The model under review builds one solid part; all positions refer to its coordinate system, in mm. Round coordinates to 2 decimals unless told otherwise and drop trailing zeros. Loops run counter-clockwise (first coordinate to the right, second up) from the corner with the lowest first, then second, coordinate; pieces in that order, holes last. Notation, with made-up numbers: (64.25, -1.5) -> (120.25, -1.5) arc R4 ccw to (120.25, 3.5) -> close; hole circle Ø2 at (14.25, 0.25). An arc over 180 degrees is marked (long way). Use a Markdown table: item, result. Add a question column.
1) Consider section A-A on z = -14.5. Give the boundary of the cut face in (x, y).
2) Consider section D-D on y = 0.4. Give the boundary of the cut face in (x, z), plus the area to 3 significant figures.
3) Consider section B-B on x = 13. Give the boundary of the cut face in (y, z).
4) Mouldability with a two-part tool opening along Z and no side actions: class faces 1 (the cylindrical face through (55.066, 1.014, -33.683)), 2 (the flat face through (17, 2, -28)) as released by +Z, released by -Z, zero draft, split by the parting line, or undercut.
5) Consider section C-C on z = 0. Give the boundary of the cut face in (x, y), plus the area to 3 significant figures.
6) Wall thickness on probe 1 along X at (y, z) = (0.4, 0); probe 2 along Z at (x, y) = (-16, 1); probe 3 along X at (y, z) = (0.55, -16.5): over which ranges is each line inside the solid? List them lowest first.
from build123d import *

# Parameters (mm, degrees)
SKETCH1_W           = 118
SKETCH1_H           = 82
BOSS_EXTRUDE1_DEPTH = 2
SKETCH2_R           = 2.45
SKETCH2_W           = 95.88
SKETCH2_H           = 65.51
SKETCH2_W_2         = 12.69
SKETCH2_H_2         = 6.85
CUT_EXTRUDE4_DEPTH  = 10
SKETCH3_R           = 1.5
CUT_EXTRUDE7_DEPTH  = 10


with BuildPart() as part:
    # Sketch1 → Boss-Extrude1 (new body)
    with BuildSketch(Plane(origin=(0, 0, 0), x_dir=(1, 0, 0), z_dir=(0, 1, 0))):
        Rectangle(SKETCH1_W, SKETCH1_H)
    extrude(amount=BOSS_EXTRUDE1_DEPTH)

    # Sketch2 → Cut-Extrude4 (cut)
    with BuildSketch(Plane(origin=(0, 2, 0), x_dir=(1, 0, 0), z_dir=(0, 1, 0))):
        with Locations(Location((53, 35, 0), (0, 0, 270))):
            Circle(SKETCH2_R)
        with Locations((-6.06, -6.245)):
            Rectangle(SKETCH2_W, SKETCH2_H)
        with Locations((-47.655, 34.575)):
            Rectangle(SKETCH2_W_2, SKETCH2_H_2)
    extrude(amount=-CUT_EXTRUDE4_DEPTH, mode=Mode.SUBTRACT)

    # Sketch3 → Cut-Extrude7 (cut)
    with BuildSketch(Plane(origin=(0, 2, 0), x_dir=(1, 0, 0), z_dir=(0, 1, 0))):
        with Locations(Location((57, 0, 0), (0, 0, 270))):
            Circle(SKETCH3_R)
        with Locations(Location((-57, 0, 0), (0, 0, 270))):
            Circle(SKETCH3_R)
    extrude(amount=-CUT_EXTRUDE7_DEPTH, mode=Mode.SUBTRACT)


solid = part.part
Result set:
| question | item | result |
|---|---|---|
| 1 | outline | (-59, 0) -> (-54, 0) -> (-54, 2) -> (-59, 2) -> close; (41.88, 0) -> (59, 0) -> (59, 2) -> (41.88, 2) -> close |
| 2 | outline | (-59, -41) -> (59, -41) -> (59, 41) -> (-59, 41) -> close; hole circle Ø3 at (-57, 0); hole (-54, -38) -> (-41.31, -38) -> (-41.31, -31.15) -> (-54, -31.15) -> close; hole (-54, -26.51) -> (41.88, -26.51) -> (41.88, 39) -> (-54, 39) -> close; hole circle Ø4.9 at (53, -35); hole circle Ø3 at (57, 0) |
| 2 | area | 3,270 mm2 |
| 3 | outline | (0, -41) -> (2, -41) -> (2, -26.51) -> (0, -26.51) -> close; (0, 39) -> (2, 39) -> (2, 41) -> (0, 41) -> close |
| 4 | face 1 | undercut |
| 4 | face 2 | zero draft |
| 5 | outline | (-59, 0) -> (-58.5, 0) -> (-58.5, 2) -> (-59, 2) -> close; (-55.5, 0) -> (-54, 0) -> (-54, 2) -> (-55.5, 2) -> close; (41.88, 0) -> (55.5, 0) -> (55.5, 2) -> (41.88, 2) -> close; (58.5, 0) -> (59, 0) -> (59, 2) -> (58.5, 2) -> close |
| 5 | area | 32.2 mm2 |
| 6 | probe 1 | -59 to -58.5, -55.5 to -54, 41.88 to 55.5, 58.5 to 59 |
| 6 | probe 2 | -41 to -26.51, 39 to 41 |
| 6 | probe 3 | -59 to -54, 41.88 to 59 |
